Can you work these out from the model? Positions are in its coordinate system, mm. A direction names the side the tool comes from. Give positions to 0.01 mm unless a question says otherwise; leave off trailing zeros. Write each loop counter-clockwise with the first axis right and the second up, starting at its lowest first coordinate (ties: lowest second). Pieces come first, ordered by that corner, then holes.
1. If I drill on probe 1 along X at (y, z) = (-122, 22); probe 2 along Y at (x, z) = (-50, 30.9); probe 3 along Y at (x, z) = (-44, 30.5), over which ranges is the centre line in solid material (lowest first)?
2. On a 3-axis mill with a long thin cutter (end or side, diameter ignored), from which of +Z, -Z, +X, -X, +Y, -Y can I reach the whole of each face in a straight line? I mean faces 1 (the flat face through (43.4, -82.5, 15.2)), 2 (the flat face through (55.61, -98.45, 14.79)), 3 (the cylindrical face through (-101.19, 50.63, 17.21)). Say none if no direction works.
3. Suppose I cut it at A-A (z = 10.5). Please give me the cut outline in (x, y).
4. Suppose I cut it at B-B (y = 0). Please give me the cut outline in (x, z).
5. I'm going to push flat-ended pins straight in: pin 1 (6 mm diameter, centred on y = 11, z = 9, fed in from -X); pin 2 (2 mm diameter, centred on y = -42.5, z = 19.5, fed in from -X); pin 3 (1 mm diameter, centred on x = 11.5, z = 31, fed in from -Y). Where does each tip first touch, or does it pass through?
6. Suppose I cut it at C-C (y = -35). Please give me the cut outline in (x, z), and give its area (3 significant figures).
7. Suppose I cut it at D-D (x = -38). Give the number of separate pieces and of enclosed holes in the cut face, and give its area (3 significant figures).
8. Thinking about a two-plate mould opening in Y: for faces 4 (the cylindrical face through (87.421, 44.313, 31.014)), 5 (the flat face through (0, -197, 32)), 6 (the cylindrical face through (105.493, 48.954, 30.986)), which applies, pulls with the +Y half, pulls with the -Y half, needs draft (parallel to the pull), parting line crosses it, or undercut?
```python
from build123d import *

# Parameters (mm, degrees)
PAD_DEPTH       = 30
PAD003_DEPTH    = 32
POCKET_DEPTH    = 30
PAD004_DEPTH    = 32
POCKET004_DEPTH = 2
POCKET001_DEPTH = 32.001
SKETCH004_W     = 160
SKETCH004_H     = 60
PAD002_DEPTH    = 30
SKETCH005_W     = 156
SKETCH005_H     = 56
PAD005_DEPTH    = 32
SKETCH009_W     = 152
SKETCH009_H     = 52
POCKET006_DEPTH = 30
SKETCH006_W     = 18
SKETCH006_H     = 12
POCKET005_DEPTH = 30
SKETCH010_W     = 20
SKETCH010_H     = 10
POCKET007_DEPTH = 5
SKETCH011_W     = 26
SKETCH011_H     = 26
POCKET008_DEPTH = 2.5


with BuildPart() as part:
    # Sketch001 → Pad (new body)
    with BuildSketch(Plane.XY):
        with BuildLine():
            ThreePointArc((0, 57.236352), (-106.486482, 50.845622), (-101.68, -55.72412))
            Line((-101.68, -55.72412), (0, -150.0248))
            Line((0, -150.0248), (101.68, -55.72412))
            ThreePointArc((101.68, -55.72412), (106.486482, 50.845622), (0, 57.236352))
        make_face()
    extrude(amount=PAD_DEPTH)

    # Sketch002 → Pad003 (join)
    with BuildSketch(Plane.XY):
        with BuildLine():
            ThreePointArc((0, 54.552727), (-104.405447, 50.160217), (-100.32, -54.257696))
            Line((-100.32, -54.257696), (0, -147.297076))
            Line((0, -147.297076), (100.32, -54.257696))
            ThreePointArc((100.32, -54.257696), (104.405447, 50.160217), (0, 54.552727))
        make_face()
    extrude(amount=PAD003_DEPTH)

    # Sketch007 → Pocket (cut)
    with BuildSketch(Plane.XY.offset(32)):
        with BuildLine():
            ThreePointArc((0, 51.807335), (-102.301889, 49.482446), (-98.96, -52.791272))
            Line((-98.96, -52.791272), (0, -144.569352))
            Line((0, -144.569352), (98.96, -52.791272))
            ThreePointArc((98.96, -52.791272), (102.301889, 49.482446), (0, 51.807335))
        make_face()
    extrude(amount=-POCKET_DEPTH, mode=Mode.SUBTRACT)

    # Sketch008 → Pad004 (join)
    with BuildSketch(Plane.XY):
        with BuildLine():
            ThreePointArc((0, 33.166248), (-88.852758, 45.721583), (-90.8, -43.992727))
            Line((-90.8, -43.992727), (0, -128.203011))
            Line((0, -128.203011), (90.8, -43.992727))
            ThreePointArc((90.8, -43.992727), (88.852758, 45.721583), (0, 33.166248))
        make_face()
    extrude(amount=PAD004_DEPTH)

    # Sketch003 → Pocket004 (cut)
    with BuildSketch(Plane.XY.offset(32)):
        with BuildLine():
            ThreePointArc((0, 29.393877), (-86.345652, 45.199486), (-89.44, -42.526302))
            Line((-89.44, -42.526302), (0, -125.475287))
            Line((0, -125.475287), (89.44, -42.526302))
            ThreePointArc((89.44, -42.526302), (86.345652, 45.199486), (0, 29.393877))
        make_face()
    extrude(amount=-POCKET004_DEPTH, mode=Mode.SUBTRACT)

    # Sketch → Pocket001 (cut, through all)
    with BuildSketch(Plane.XY.offset(32)):
        with BuildLine():
            ThreePointArc((0, 25.21904), (-83.671135, 44.74656), (-88.08, -41.059878))
            Line((-88.08, -41.059878), (0, -122.747563))
            Line((0, -122.747563), (88.08, -41.059878))
            ThreePointArc((88.08, -41.059878), (83.671135, 44.74656), (0, 25.21904))
        make_face()
    extrude(amount=-POCKET001_DEPTH, mode=Mode.SUBTRACT)

    # Sketch004 → Pad002 (join)
    with BuildSketch(Plane.XY):
        with Locations((0, -170)):
            Rectangle(SKETCH004_W, SKETCH004_H)
    extrude(amount=PAD002_DEPTH)

    # Sketch005 → Pad005 (join)
    with BuildSketch(Plane.XY):
        with Locations((0, -170)):
            Rectangle(SKETCH005_W, SKETCH005_H)
    extrude(amount=PAD005_DEPTH)

    # Sketch009 → Pocket006 (cut)
    with BuildSketch(Plane.XY.offset(32)):
        with Locations((0, -170)):
            Rectangle(SKETCH009_W, SKETCH009_H)
    extrude(amount=-POCKET006_DEPTH, mode=Mode.SUBTRACT)

    # Sketch006 → Pocket005 (cut)
    with BuildSketch(Plane.XY.offset(32)):
        with Locations((0, -142.076699)):
            Rectangle(SKETCH006_W, SKETCH006_H)
    extrude(amount=-POCKET005_DEPTH, mode=Mode.SUBTRACT)

    # Sketch010 → Pocket007 (cut, symmetric)
    with BuildSketch(Plane.YZ.offset(80)):
        with Locations((-168.343253, 19)):
            Rectangle(SKETCH010_W, SKETCH010_H)
    extrude(amount=POCKET007_DEPTH, both=True, mode=Mode.SUBTRACT)

    # Sketch011 → Pocket008 (cut, symmetric)
    with BuildSketch(Plane.XY):
        with Locations((-41, -169.18593)):
            Rectangle(SKETCH011_W, SKETCH011_H)
        with Locations((0, -169.18593)):
            Rectangle(SKETCH011_W, SKETCH011_H)
        with Locations((41, -169.18593)):
            Rectangle(SKETCH011_W, SKETCH011_H)
    extrude(amount=POCKET008_DEPTH, both=True, mode=Mode.SUBTRACT)


solid = part.part
```
Checks:
1. probe 1: x = -30.22 to -24.34, -6.69 to -0.81, 0.81 to 6.69, 24.34 to 30.22
1. probe 2: y = -198 to -196, -144 to -142, -100.93 to -98.2, -81.83 to -79.1, 58 to 60, 72 to 74
1. probe 3: y = -198 to -196, -144 to -142, -106.49 to -103.76, -87.4 to -84.67, 57.69 to 59.7, 71.75 to 73.76
2. face 1: +Z, -Z
2. face 2: +Z, -Z, +X
2. face 3: +Z
3. outline: (-101.68, -55.72) - (-10.81, -140) - (-80, -140) - (-80, -200) - (80, -200) - (80, -140) - (10.81, -140) - (101.68, -55.72) arc R76 ccw to (0, 57.24) arc R76 ccw to start; (-90.8, -43.99) - (0, -128.2) - (90.8, -43.99) arc R60 ccw (long way) to (0, 33.17) arc R60 ccw (long way) to start; hole (-98.96, -52.79) - (-9, -136.22) - (-9, -144) - (-76, -144) - (-76, -196) - (76, -196) - (76, -144) - (9, -144) - (9, -136.22) - (98.96, -52.79) arc R72 ccw (long way) to (0, 51.81) arc R72 ccw (long way) to start; hole (-88.08, -41.06) - (0, -122.75) - (88.08, -41.06) arc R56 ccw (long way) to (0, 25.22) arc R56 ccw (long way) to start
4. outline: (-126, 0) - (-106, 0) - (-106, 30) - (-108, 30) - (-108, 32) - (-110, 32) - (-110, 2) - (-122, 2) - (-122, 32) - (-124, 32) - (-124, 30) - (-126, 30) - close; (106, 0) - (126, 0) - (126, 30) - (124, 30) - (124, 32) - (122, 32) - (122, 2) - (110, 2) - (110, 32) - (108, 32) - (108, 30) - (106, 30) - close
5. pin 1: stops at x = -125.58
5. pin 2: stops at x = -113.67
5. pin 3: stops at y = -198
6. outline: (-117.46, 0) - (-93.71, 0) - (-93.71, 30) - (-96.25, 30) - (-96.25, 32) - (-98.73, 32) - (-98.73, 2) - (-112.92, 2) - (-112.92, 32) - (-115.2, 32) - (-115.2, 30) - (-117.46, 30) - close; (93.71, 0) - (117.46, 0) - (117.46, 30) - (115.2, 30) - (115.2, 32) - (112.92, 32) - (112.92, 2) - (98.73, 2) - (98.73, 32) - (96.25, 32) - (96.25, 30) - (93.71, 30) - close
6. area: 649 mm2
7. separate pieces: 4
7. enclosed holes: 0
7. area: 948 mm2
8. face 4: undercut
8. face 5: needs draft
8. face 6: parting line crosses it
